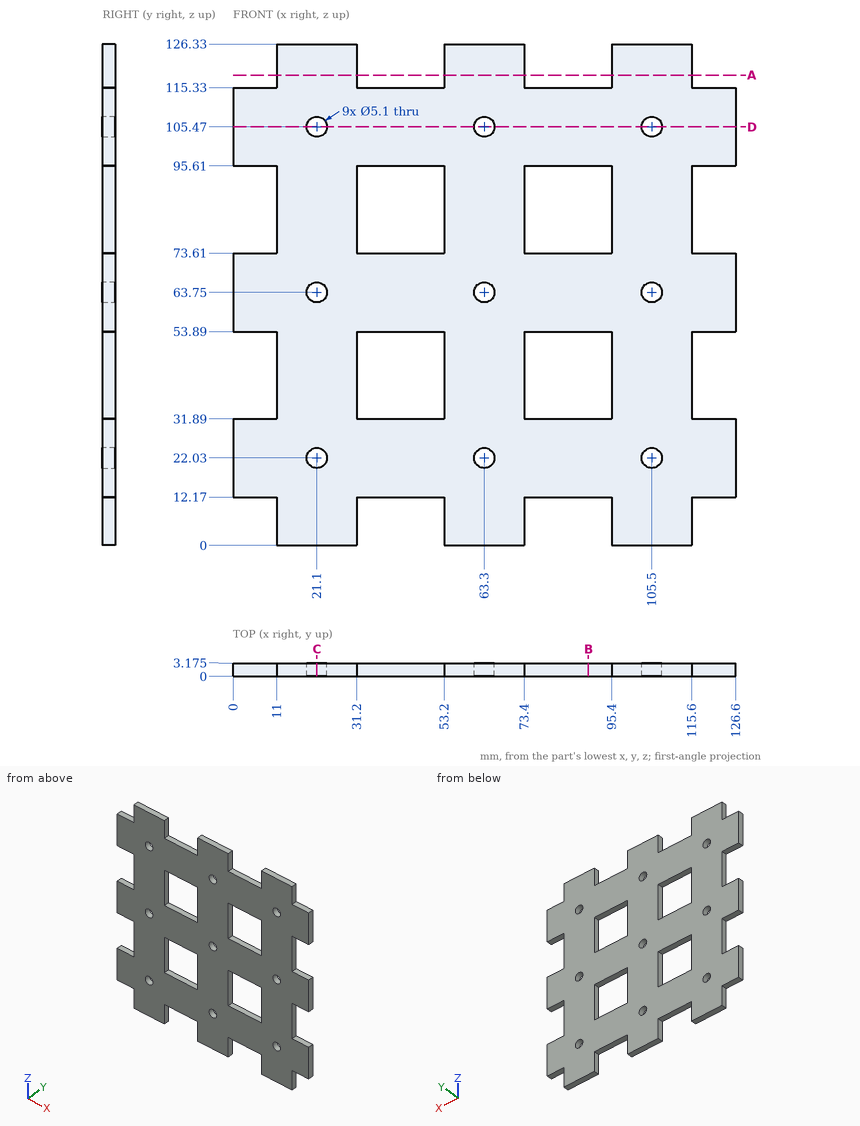
Design review of the part shown in the three views and the two pictorial views. Dimensions are in mm from the part's minimum x, y and z. Round coordinates to 2 decimals unless told otherwise and drop trailing zeros. Write each loop counter-clockwise with the first axis right and the second up, starting at its lowest first coordinate (ties: lowest second). Pieces come first, ordered by that corner, then holes. Notation, with made-up numbers: M 54.25,6.25 L 87.25,6.25 A8 ccw 87.25,18.25 Z; hole C -14.5,-31 d4. An arc over 180 degrees is marked long. Use a Markdown table: item, result. Add a question column.
Q1. We need section D-D, the plane z = 105.47. State the section outline as (x, y) points (3 decimals).
Q2. We need section C-C, the plane x = 21.1. State the section outline as (y, z) points (3 decimals), plus the area to 3 significant figures.
Q3. We need section B-B, the plane x = 89.5. State the section outline as (y, z) points (3 decimals), plus the area to 3 significant figures.
Q4. To check wall thickness, follow line 1 (X direction, y = 1.15, z = 84); line 2 (X direction, y = 1.7, z = 105.47); line 3 (Z direction, x = 105.5, y = 1.9). State the ranges of each line that lie inside material, in increasing order.
Q5. Insertion check: pin 1 (1 mm diameter, centred on x = 89, y = 1.5, fed in from +Z); pin 2 (1 mm diameter, centred on y = 1, z = 89, fed in from -X); pin 3 (12 mm diameter, centred on x = 60.5, z = 31.5, fed in from -Y); pin 4 (1.6 mm diameter, centred on y = 2.5, z = 8, fed in from +X). Each pin has a flat end and moves straight along its axis. Give the tip position at first contact, or say it passes through.
Q6. We need section A-A, the plane z = 118.5. State the section outline as (x, y) points (3 decimals).
Findings below:
| question | item | result |
|---|---|---|
| 1 | outline | M 0,0 L 18.55,0 L 18.55,3.175 L 0,3.175 Z; M 23.65,0 L 60.75,0 L 60.75,3.175 L 23.65,3.175 Z; M 65.85,0 L 102.95,0 L 102.95,3.175 L 65.85,3.175 Z; M 108.05,0 L 126.6,0 L 126.6,3.175 L 108.05,3.175 Z |
| 2 | outline | M 0,0 L 3.175,0 L 3.175,19.48 L 0,19.48 Z; M 0,24.58 L 3.175,24.58 L 3.175,61.2 L 0,61.2 Z; M 0,66.3 L 3.175,66.3 L 3.175,102.92 L 0,102.92 Z; M 0,108.02 L 3.175,108.02 L 3.175,126.33 L 0,126.33 Z |
| 2 | area | 353 mm² |
| 3 | outline | M 0,12.17 L 3.175,12.17 L 3.175,31.89 L 0,31.89 Z; M 0,53.89 L 3.175,53.89 L 3.175,73.61 L 0,73.61 Z; M 0,95.61 L 3.175,95.61 L 3.175,115.33 L 0,115.33 Z |
| 3 | area | 188 mm² |
| 4 | line 1 | x = 11 to 31.2, 53.2 to 73.4, 95.4 to 115.6 |
| 4 | line 2 | x = 0 to 18.55, 23.65 to 60.75, 65.85 to 102.95, 108.05 to 126.6 |
| 4 | line 3 | z = 0 to 19.48, 24.58 to 61.2, 66.3 to 102.92, 108.02 to 126.33 |
| 5 | pin 1 | stops at z = 115.33 |
| 5 | pin 2 | stops at x = 11 |
| 5 | pin 3 | stops at y = 0 |
| 5 | pin 4 | stops at x = 115.6 |
| 6 | outline | M 11,0 L 31.2,0 L 31.2,3.175 L 11,3.175 Z; M 53.2,0 L 73.4,0 L 73.4,3.175 L 53.2,3.175 Z; M 95.4,0 L 115.6,0 L 115.6,3.175 L 95.4,3.175 Z |
